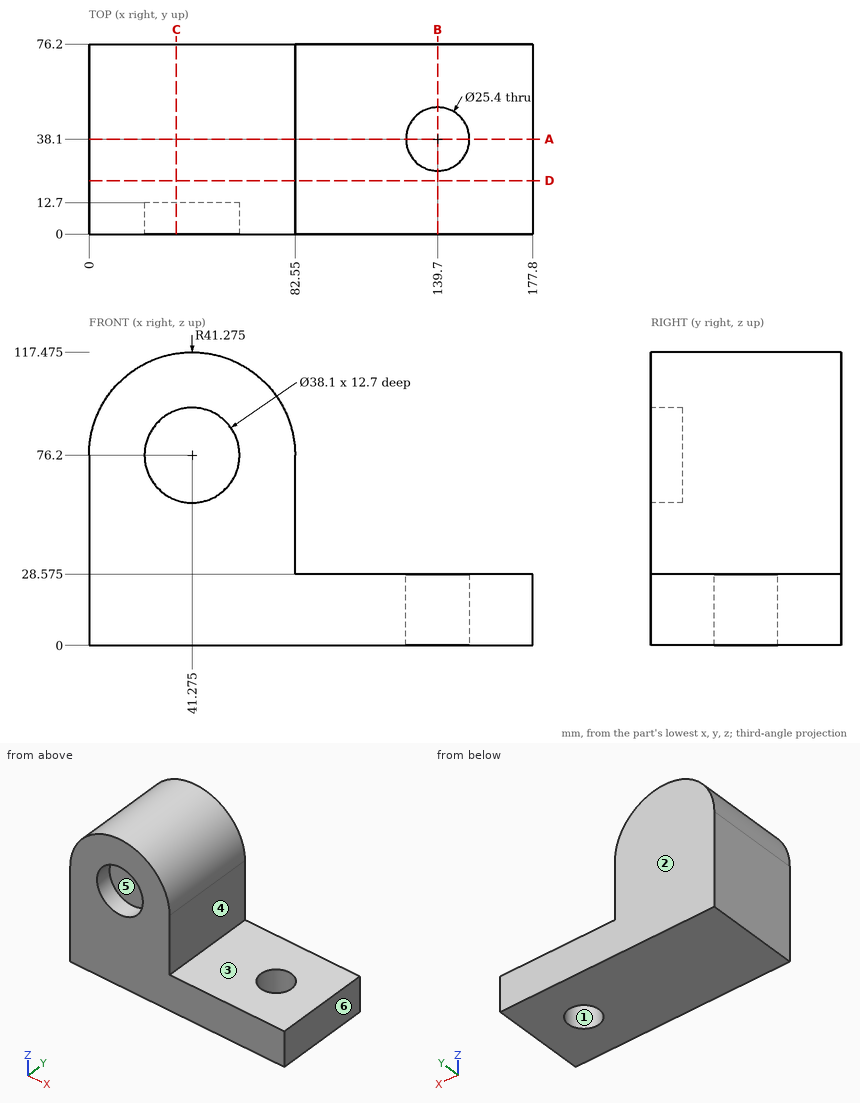
Check sheet for the drawn part. Datum: minimum x, y, z corner. Units: mm. A direction names the side the tool comes from. Give positions to 0.01 mm unless a question says otherwise; leave off trailing zeros. Order: outer loops, then holes, each group sorted by start corner. A loop starts at its lowest first (then second) coordinate and runs counter-clockwise, first axis right, second up. Notation, with made-up numbers: (28.5, 3) - (37.5, 3) arc R24 ccw to (37.5, 33) - close; hole circle Ø11 at (-36.75, -36). An arc over 180 degrees is marked (long way). Write item = value, one per line. Start each with the question number.
1) Section check B-B (x = 139.7). Enter the section's corners in (y, z) (3 decimals), then the cut area to 3 significant figures.
2) Scan lines: L1, parallel to X at y = 38, z = 15; L2, parallel to Y at x = 139.7, z = 18.5; L3, parallel to X at y = 4, z = 76. Record each from-to range of solid material in increasing order.
3) Section check C-C (x = 35). Enter the section's corners in (y, z), then the cut area to 3 significant figures.
4) Section check A-A (y = 38.1). Enter the section's corners in (x, z) (3 decimals).
5) Draft check along Y on the marked faces 1, 2 and 3. Enter one of: released by +Y, released by -Y, zero draft, split by the parting line, or undercut.
6) Gauge pin test, flat ends, axial feed: pin 1 Ø23 at (x, y) = (139.7, 38.1) entering from -Z; pin 2 Ø2 at (x, y) = (153.5, 32) entering from +Z (3 decimals); pin 3 Ø24 at (y, z) = (51.5, 41.5) entering from +X; pin 4 Ø10 at (y, z) = (25, 78.5) entering from +X. Record the tip position at first contact, or that the pin passes through.
7) Access from +Z, -Z, +X, -X, +Y, -Y to the whole of each face (thin tool, end or side, straight path). Record for the marked faces 4, 5 and 6.
8) Section check D-D (y = 21.5). Enter the section's corners in (x, z) (3 decimals).
Geometry check:
q1.outline = (0, 0) - (25.4, 0) - (25.4, 28.575) - (0, 28.575) - close; (50.8, 0) - (76.2, 0) - (76.2, 28.575) - (50.8, 28.575) - close
q1.area = 1,450 mm2
q2.L1 = 0 to 127, 152.4 to 177.8
q2.L2 = 0 to 25.4, 50.8 to 76.2
q2.L3 = 0 to 22.23, 60.32 to 82.55
q3.outline = (0, 0) - (76.2, 0) - (76.2, 117) - (0, 117) - (0, 94.19) - (12.7, 94.19) - (12.7, 58.21) - (0, 58.21) - close
q3.area = 8,460 mm2
q4.outline = (0, 0) - (127, 0) - (127, 28.575) - (82.55, 28.575) - (82.55, 76.2) arc R41.275 ccw to (0, 76.2) - close; (152.4, 0) - (177.8, 0) - (177.8, 28.575) - (152.4, 28.575) - close
q5.face_1 = undercut
q5.face_2 = released by +Y
q5.face_3 = zero draft
q6.pin_1 = through
q6.pin_2 = 28.575
q6.pin_3 = 82.55
q6.pin_4 = 82.55
q7.face_4 = +Z, +X, +Y, -Y
q7.face_5 = -Y
q7.face_6 = +Z, -Z, +X, +Y, -Y
q8.outline = (0, 0) - (177.8, 0) - (177.8, 28.575) - (82.55, 28.575) - (82.55, 76.2) arc R41.275 ccw to (0, 76.2) - close
